from build123d import *

# Parameters (mm, degrees)
SKETCH_1_W          = 190
SKETCH_1_H          = 52
SKETCH_1_R          = 1.6
SKETCH_1_W_2        = 75
SKETCH_1_H_2        = 36
EXTRUDE_1_DEPTH     = 2
CUT_EXTRUDE_1_DEPTH = 2
EXTRUDE_1_2_DEPTH   = 2
FILLET_1_R          = 1.5


with BuildPart() as part:
    # 草图1 → Extrude 1 (new body)
    with BuildSketch(Plane(origin=(0, 0, 0), x_dir=(1, 0, 0), z_dir=(0, 1, 0))):
        Rectangle(SKETCH_1_W, SKETCH_1_H)
        with Locations(Location((91, -10, 0), (0, 0, 270))):
            Circle(SKETCH_1_R, mode=Mode.SUBTRACT)
        with Locations(Location((91, 10, 0), (0, 0, 270))):
            Circle(SKETCH_1_R, mode=Mode.SUBTRACT)
        with Locations(Location((-91, 10, 0), (0, 0, 270))):
            Circle(SKETCH_1_R, mode=Mode.SUBTRACT)
        with Locations(Location((-91, -10, 0), (0, 0, 270))):
            Circle(SKETCH_1_R, mode=Mode.SUBTRACT)
        with Locations(Location((41.5, -20, 0), (0, 0, 270))):
            Circle(SKETCH_1_R, mode=Mode.SUBTRACT)
        with Locations(Location((-41.5, -20, 0), (0, 0, 270))):
            Circle(SKETCH_1_R, mode=Mode.SUBTRACT)
        with Locations(Location((-41.5, 20, 0), (0, 0, 270))):
            Circle(SKETCH_1_R, mode=Mode.SUBTRACT)
        with Locations(Location((41.5, 20, 0), (0, 0, 270))):
            Circle(SKETCH_1_R, mode=Mode.SUBTRACT)
        Rectangle(SKETCH_1_W_2, SKETCH_1_H_2, mode=Mode.SUBTRACT)
    extrude(amount=EXTRUDE_1_DEPTH)

    # 草图2 → 切除-拉伸1 (cut)
    with BuildSketch(Plane(origin=(0, 2, 0), x_dir=(1, 0, 0), z_dir=(0, 1, 0))):
        Polygon((95, 13.207136478), (37.560055456, 26), (95, 26), align=None)
        Polygon((37.560055456, -26), (95, -26), (95, -13.207136478), align=None)
        Polygon((-95, -26), (-95, -13.207136478), (-37.560055456, -26), align=None)
        Polygon((-95, 26), (-95, 13.207136478), (-37.560055456, 26), align=None)
        Polygon((45.5, 19.109131207), (45.5, -19.109131207), (87, -9.866367475), (87, 9.866367475), align=None)
        Polygon((-87, -9.866367475), (-87, 9.866367475), (-45.5, 19.109131207), (-45.5, -19.109131207), align=None)
    extrude(amount=-CUT_EXTRUDE_1_DEPTH, mode=Mode.SUBTRACT)

    # 草图3 → Extrude 1 2 (add)
    with BuildSketch(Plane(origin=(0, 2, 0), x_dir=(1, 0, 0), z_dir=(0, 1, 0))):
        Polygon((-44.355051898, -17.46928553), (-85.855051898, 11.506213152), (-88.144948102, 8.226521799), (-46.644948102, -20.748976883), align=None)
        Polygon((36.634537865, 19.803046115), (-38.365462135, -16.196953885), (-36.634537865, -19.803046115), (38.365462135, 16.196953885), align=None)
        Polygon((-38.365462135, 16.196953885), (36.634537865, -19.803046115), (38.365462135, -16.196953885), (-36.634537865, 19.803046115), align=None)
        Polygon((46.644948102, -20.748976883), (88.144948102, 8.226521799), (85.855051898, 11.506213152), (44.355051898, -17.46928553), align=None)
    extrude(amount=-EXTRUDE_1_2_DEPTH)

    # 圆角1
    fillet_1_edges = [part.edges().sort_by_distance(p)[0] for p in [
        (-87, 1, 9.866367475),
        (-45.5, 1, -19.109131207),
        (95, 1, -13.207136478),
        (37.560055456, 1, -26),
        (-45.5, 1, 16.669877284),
        (-87, 1, -7.427113552),
        (-50.630005448, 1, 17.966590766),
        (-84.351291466, 1, -10.456280419),
        (32.878191792, 1, 18),
        (-32.878191792, 1, 18),
        (-37.5, 1, -15.78153206),
        (-37.5, 1, 15.78153206),
        (-32.878191792, 1, -18),
        (32.878191792, 1, -18),
        (37.5, 1, 15.78153206),
        (37.5, 1, -15.78153206),
        (0, 1, -2.21846794),
        (0, 1, 2.21846794),
        (4.621808208, 1, 0),
        (-4.621808208, 1, 0),
        (45.5, 1, 16.669877284),
        (50.630005448, 1, 17.966590766),
        (87, 1, -7.427113552),
        (84.351291466, 1, -10.456280419),
        (45.5, 1, -19.109131207),
        (87, 1, 9.866367475),
        (-37.560055456, 1, -26),
        (-95, 1, -13.207136478),
        (-37.560055456, 1, 26),
        (-95, 1, 13.207136478),
        (37.560055456, 1, 26),
        (95, 1, 13.207136478),
    ]]
    fillet(fillet_1_edges, radius=FILLET_1_R)


solid = part.part
The listing builds one solid part. Answer for the finished solid, in the listing's coordinates (mm). Give positions to 0.01 mm unless a question says otherwise; leave off trailing zeros. Write each loop counter-clockwise with the first axis right and the second up, starting at its lowest first coordinate (ties: lowest second). Pieces come first, ordered by that corner, then holes.
Item 1: Flat-ended cylindrical pins translate along their axes: P1, Ø4, axis at x = 41.5, z = -20, coming from the -Y side; P2, Ø1.9, axis at x = -91, z = -10, coming from the -Y side. Find the tip coordinate at first contact, or state that the pin passes through.
Item 2: Find the intervals of material crossed by line 1 along Z through (x, y) = (-91, 1.4); line 2 along Z through (x, y) = (6, 0.5); line 3 along Z through (x, y) = (-24.5, 0.65), in increasing order.
Item 3: Section D-D, the plane x = -49.5 is taken. Write down the section's boundary in (y, z).
Item 4: Determine the mould class of faces 1 (the flat face through (-66.17, 1.01, -19.63)), 2 (the flat face through (13.61, 1.01, 8.75)), 3 (the flat face through (66.17, 1.01, 19.63)) for opening direction X: released by +X, released by -X, zero draft, split by the parting line, or undercut.
Item 5: Section A-A, the plane x = -18.5 is taken. Write down the section's boundary in (y, z), plus the area to 3 significant figures.
Item 6: Section C-C, the plane x = 91 is taken. Write down the section's boundary in (y, z), plus the area to 3 significant figures.
Item 7: Section B-B, the plane z = 20 is taken. Write down the section's boundary in (x, y), plus the area to 3 significant figures.
Completed:
1. P1: stops at y = 0
1. P2: passes through
2. line 1: z = -14.1 to -11.6, -8.4 to 8.4, 11.6 to 14.1
2. line 2: z = -26 to -18, -5.1 to 5.1, 18 to 26
2. line 3: z = -26 to -18, -13.98 to -9.54, 9.54 to 13.98, 18 to 26
3. outline: (0, -23.34) - (2, -23.34) - (2, -18.22) - (0, -18.22) - close; (0, 13.88) - (2, 13.88) - (2, 23.34) - (0, 23.34) - close
4. face 1: released by -X
4. face 2: undercut
4. face 3: released by +X
5. outline: (0, -26) - (2, -26) - (2, -18) - (0, -18) - close; (0, -11.1) - (2, -11.1) - (2, -6.66) - (0, -6.66) - close; (0, 6.66) - (2, 6.66) - (2, 11.1) - (0, 11.1) - close; (0, 18) - (2, 18) - (2, 26) - (0, 26) - close
5. area: 49.7 mm2
6. outline: (0, -14.1) - (2, -14.1) - (2, -11.6) - (0, -11.6) - close; (0, -8.4) - (2, -8.4) - (2, 8.4) - (0, 8.4) - close; (0, 11.6) - (2, 11.6) - (2, 14.1) - (0, 14.1) - close
6. area: 43.6 mm2
7. outline: (-64.5, 0) - (-43.1, 0) - (-43.1, 2) - (-64.5, 2) - close; (-39.9, 0) - (39.9, 0) - (39.9, 2) - (-39.9, 2) - close; (43.1, 0) - (64.5, 0) - (64.5, 2) - (43.1, 2) - close
7. area: 245 mm2
